```python
from build123d import *

# Parameters (mm, degrees)
CROQUIS1_W              = 254.7
CROQUIS1_H              = 6.25
SALIENTE_EXTRUIR1_DEPTH = 3.125
CROQUIS2_R              = 1.5
CORTAR_EXTRUIR1_DEPTH   = 20
CROQUIS3_R              = 1.5
CORTAR_EXTRUIR2_DEPTH   = 30


with BuildPart() as part:
    # Croquis1 → Saliente-Extruir1 (new, symmetric)
    with BuildSketch(Plane(origin=(0, 0, 0), x_dir=(0, 0, -1), z_dir=(1, 0, 0))):
        Rectangle(CROQUIS1_W, CROQUIS1_H)
    extrude(amount=SALIENTE_EXTRUIR1_DEPTH, both=True)

    # Croquis2 → Cortar-Extruir1 (cut, symmetric)
    with BuildSketch(Plane(origin=(3.125, 0, 0), x_dir=(0, 0, -1), z_dir=(1, 0, 0))):
        with Locations(Location((-122.975, 0, 0), (0, 0, 180))):
            Circle(CROQUIS2_R)
        with Locations(Location((122.975, 0, 0), (0, 0, 180))):
            Circle(CROQUIS2_R)
    extrude(amount=CORTAR_EXTRUIR1_DEPTH, both=True, mode=Mode.SUBTRACT)

    # Croquis3 → Cortar-Extruir2 (cut, symmetric)
    with BuildSketch(Plane.XZ.offset(3.125)):
        with Locations(Location((0, 115.475, 0), (0, 0, 270))):
            Circle(CROQUIS3_R)
        with Locations(Location((0, -115.475, 0), (0, 0, 270))):
            Circle(CROQUIS3_R)
        with Locations(Location((0, 0, 0), (0, 0, 270))):
            Circle(CROQUIS3_R)
    extrude(amount=CORTAR_EXTRUIR2_DEPTH, both=True, mode=Mode.SUBTRACT)


solid = part.part
```
The listing builds one solid part. Answer for the finished solid, in the listing's coordinates (mm). Give positions to 0.01 mm unless a question says otherwise; leave off trailing zeros. Order: outer loops, then holes, each group sorted by start corner. A loop starts at its lowest first (then second) coordinate and runs counter-clockwise, first axis right, second up. Notation, with made-up numbers: (-16.5, -18.75) -> (-0.5, -18.75) arc R10 ccw to (-0.5, -10.75) -> close; hole circle Ø8 at (71, 0.5). An arc over 180 degrees is marked (long way). Answer as CSV lines item,"result". Start each with the question number.
Q1. A cutting plane is placed at A-A (y = 0). Determine the outline of the cut face in (x, z) (3 decimals), then the cut area to 3 significant figures.
Q2. A cutting plane is placed at B-B (x = 0). Determine the outline of the cut face in (y, z) (3 decimals), then the cut area to 3 significant figures.
Q3. Find the intervals of material crossed by L1, parallel to Z at x = 2, y = -0.25; L2, parallel to Z at x = 0.25, y = 2.5; L3, parallel to X at y = 0.75, z = 0 (3 decimals), in increasing order.
Results found:
1,outline,"(-3.125, -127.35) -> (3.125, -127.35) -> (3.125, -124.475) -> (-3.125, -124.475) -> close; (-3.125, -121.475) -> (3.125, -121.475) -> (3.125, 121.475) -> (-3.125, 121.475) -> close; (-3.125, 124.475) -> (3.125, 124.475) -> (3.125, 127.35) -> (-3.125, 127.35) -> close; hole circle Ø3 at (0, -115.475); hole circle Ø3 at (0, 0); hole circle Ø3 at (0, 115.475)"
1,area,"1,530 mm2"
2,outline,"(-3.125, -127.35) -> (3.125, -127.35) -> (3.125, -116.975) -> (-3.125, -116.975) -> close; (-3.125, -113.975) -> (3.125, -113.975) -> (3.125, -1.5) -> (-3.125, -1.5) -> close; (-3.125, 1.5) -> (3.125, 1.5) -> (3.125, 113.975) -> (-3.125, 113.975) -> close; (-3.125, 116.975) -> (3.125, 116.975) -> (3.125, 127.35) -> (-3.125, 127.35) -> close; hole circle Ø3 at (0, -122.975); hole circle Ø3 at (0, 122.975)"
2,area,"1,520 mm2"
3,L1,"-127.35 to -124.45, -121.5 to 121.5, 124.45 to 127.35"
3,L2,"-127.35 to -116.95, -114 to -1.48, 1.48 to 114, 116.95 to 127.35"
3,L3,"-3.125 to -1.5, 1.5 to 3.125"
